```python
from build123d import *

# Parameters (mm, degrees)
SKETCH_1_R          = 6.4
EXTRUDE_1_DEPTH     = 4
SKETCH_2_R          = 7.15
EXTRUDE_2_DEPTH     = 1.5
SKETCH_3_R          = 5.9
EXTRUDE_3_DEPTH     = 11
SKETCH_4_R          = 4.9
EXTRUDE_4_DEPTH     = 3.5
SKETCH_5_R          = 5
CUT_EXTRUDE_1_DEPTH = 15
SKETCH_6_R          = 1.5
CUT_EXTRUDE_2_DEPTH = 5


with BuildPart() as part:
    # ｽｹｯﾁ1 → ﾎﾞｽ - 押し出し1 (new body)
    with BuildSketch(Plane(origin=(0, 0, 0), x_dir=(1, 0, 0), z_dir=(0, 1, 0))):
        with Locations(Location((0, 0, 0), (0, 0, 270))):
            Circle(SKETCH_1_R)
    extrude(amount=EXTRUDE_1_DEPTH)

    # ｽｹｯﾁ2 → ﾎﾞｽ - 押し出し2 (add)
    with BuildSketch(Plane(origin=(0, 4, 0), x_dir=(1, 0, 0), z_dir=(0, 1, 0))):
        with Locations(Location((0, 0, 0), (0, 0, 270))):
            Circle(SKETCH_2_R)
    extrude(amount=EXTRUDE_2_DEPTH)

    # ｽｹｯﾁ3 → ﾎﾞｽ - 押し出し3 (add)
    with BuildSketch(Plane(origin=(0, 5.5, 0), x_dir=(1, 0, 0), z_dir=(0, 1, 0))):
        with Locations(Location((0, 0, 0), (0, 0, 270))):
            Circle(SKETCH_3_R)
    extrude(amount=EXTRUDE_3_DEPTH)

    # ｽｹｯﾁ4 → ﾎﾞｽ - 押し出し4 (add)
    with BuildSketch(Plane(origin=(0, 16.5, 0), x_dir=(1, 0, 0), z_dir=(0, 1, 0))):
        with Locations(Location((0, 0, 0), (0, 0, 270))):
            Circle(SKETCH_4_R)
    extrude(amount=EXTRUDE_4_DEPTH)

    # ｽｹｯﾁ5 → ｶｯﾄ - 押し出し1 (cut)
    with BuildSketch(Plane(origin=(0, 0, 0), x_dir=(-1, 0, 0), z_dir=(0, -1, 0))):
        with Locations(Location((0, 0, 0), (0, 0, 90))):
            Circle(SKETCH_5_R)
    extrude(amount=-CUT_EXTRUDE_1_DEPTH, mode=Mode.SUBTRACT)

    # ｽｹｯﾁ6 → ｶｯﾄ - 押し出し2 (cut)
    with BuildSketch(Plane(origin=(0, 20, 0), x_dir=(1, 0, 0), z_dir=(0, 1, 0))):
        with Locations(Location((0, 0, 0), (0, 0, 270))):
            Circle(SKETCH_6_R)
    extrude(amount=-CUT_EXTRUDE_2_DEPTH, mode=Mode.SUBTRACT)


solid = part.part
```
CAD build for the part. Positions are in the model's coordinates, mm. A direction names the side the tool comes from. Give positions to 0.01 mm unless a question says otherwise; leave off trailing zeros. Order: outer loops, then holes, each group sorted by start corner. A loop starts at its lowest first (then second) coordinate and runs counter-clockwise, first axis right, second up.
(1) Mould opens along Z. For faces 1 (the cylindrical face through (-5.76, 10.92, -1.28)), 2 (the cylindrical face through (0.45, 17.54, 1.43)), 3 (the flat face through (6, 5.5, 1)) say: released by +Z, released by -Z, zero draft, split by the parting line, or undercut.
(2) Saw through at C-C, the plane y = 9.5. Give the cut face in (x, z).
(3) Tool access for faces 4 (the cylindrical face through (7.09, 4.74, -0.93)), 5 (the cylindrical face through (-4.88, 7.4, 1.08)), 6 (the cylindrical face through (1.472, 18.226, 4.674)): list every direction of +Z, -Z, +X, -X, +Y, -Y with a clear straight run to the whole face (end or side of a thin tool).
(4) Saw through at A-A, the plane z = 0. Give the cut face in (x, y), then the cut area to 4 significant figures.
(5) Drill centre lines: L1, parallel to X at y = 3.75, z = 0; L2, parallel to X at y = 8.25, z = 0; L3, parallel to Y at x = -4.5, z = 3. Where is each one in solid material? Low to high.
(6) Flat gauge pins, fed straight in: pin 1 (6 mm diameter, centred on y = 17, z = -2, fed in from +X); pin 2 (8 mm diameter, centred on x = 0, z = 0, fed in from -Y); pin 3 (2 mm diameter, centred on y = 7, z = -3.5, fed in from +X). Where does each tip first touch, or does it go through?
(7) Saw through at D-D, the plane z = 5.5. Give the cut face in (x, y).
(8) Saw through at B-B, the plane x = 0. Give the cut face in (y, z), then the cut area to 4 significant figures.
Results found:
1. face 1: split by the parting line
1. face 2: undercut
1. face 3: zero draft
2. outline: circle Ø11.8 at (0, 0); hole circle Ø10 at (0, 0)
3. face 4: +Y, -Y
3. face 5: -Y
3. face 6: +Y
4. outline: (-7.15, 4) - (-6.4, 4) - (-6.4, 0) - (-5, 0) - (-5, 15) - (-1.5, 15) - (-1.5, 20) - (-4.9, 20) - (-4.9, 16.5) - (-5.9, 16.5) - (-5.9, 5.5) - (-7.15, 5.5) - close; (1.5, 15) - (5, 15) - (5, 0) - (6.4, 0) - (6.4, 4) - (7.15, 4) - (7.15, 5.5) - (5.9, 5.5) - (5.9, 16.5) - (4.9, 16.5) - (4.9, 20) - (1.5, 20) - close
4. area: 71.75 mm2
5. L1: x = -6.4 to -5, 5 to 6.4
5. L2: x = -5.9 to -5, 5 to 5.9
5. L3: y = 0 to 16.5
6. pin 1: stops at x = 5.9
6. pin 2: stops at y = 15
6. pin 3: stops at x = 5.34
7. outline: (-4.57, 4) - (-3.27, 4) - (-3.27, 0) - (3.27, 0) - (3.27, 4) - (4.57, 4) - (4.57, 5.5) - (2.14, 5.5) - (2.14, 16.5) - (-2.14, 16.5) - (-2.14, 5.5) - (-4.57, 5.5) - close
8. outline: (0, -6.4) - (4, -6.4) - (4, -7.15) - (5.5, -7.15) - (5.5, -5.9) - (16.5, -5.9) - (16.5, -4.9) - (20, -4.9) - (20, -1.5) - (15, -1.5) - (15, -5) - (0, -5) - close; (0, 5) - (15, 5) - (15, 1.5) - (20, 1.5) - (20, 4.9) - (16.5, 4.9) - (16.5, 5.9) - (5.5, 5.9) - (5.5, 7.15) - (4, 7.15) - (4, 6.4) - (0, 6.4) - close
8. area: 71.75 mm2
